Here's how the part is built. I have some questions about the finished solid (model axes, mm). Round coordinates to 2 decimals unless told otherwise and drop trailing zeros. Loops run counter-clockwise (first coordinate to the right, second up) from the corner with the lowest first, then second, coordinate; pieces in that order, holes last. Notation, with made-up numbers: M 83,63.5 L 121,63.5 A22 cw 121,94.5 Z; hole C 58,51 d8. An arc over 180 degrees is marked long. Write each question's results on one line, items separated by ' | '. Start each with the question number.
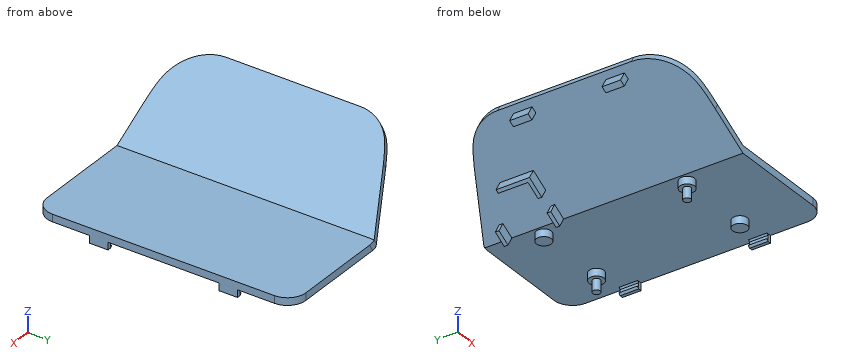
Autodesk Inventor part; units mm, degrees
ref_plane "YZ Plane" through (0, 0, 0) normal (1, 0, 0) x (0, 1, 0)
ref_plane "XZ Plane" through (0, 0, 0) normal (0, 1, 0) x (-1, 0, 0)
ref_plane "XY Plane" through (0, 0, 0) normal (0, 0, 1) x (1, 0, 0)
sketch "スケッチ1" plane through (0, 0, 0) normal (0, 0, 1) x (1, 0, 0)
  line L0 (0, 0) -> (-32, 0)
  line L1 (-32, 0) -> (-32, -70)
  line L2 (-32, -70) -> (0, -70)
  line L3 (0, -70) -> (0, 0)
  dimension "d0" = 32
  dimension "d1" = 70
extrude "押し出し1" add sketch "スケッチ1" along normal blind 2
sketch "スケッチ2" plane through (-32, -70, 0) normal (0, -1, 0) x (1, 0, 0)
  line L0 (0, 0) -> (32, 0)
  line L1 (32, 0) -> (32, 2)
  line L2 (0, 2) -> (32, 2)
  line L3 (0, 0) -> (0, 2)
  line L4 (0, 0) -> (-25.9808, 15)
  line L5 (-25.9808, 15) -> (-25.1147, 16.5)
  line L6 (-25.1147, 16.5) -> (0, 2)
  point P0 (32, 0)
  dimension "d4" = 30
  dimension "d5" = 150
extrude "押し出し2" add sketch "スケッチ2" against normal blind 70 contours L4 L5 L6 L3
sketch "スケッチ3" plane through (0, 0, 0) normal (0, 0, -1) x (-1, 0, 0)
  line L0 (0, 0) -> (32, 0)
  line L1 (32, 0) -> (57.9808, -12.115)
  line L2 (32, 0) -> (57.9808, 0)
  line L3 (57.9808, -70) -> (57.9808, 0)
  dimension "d8" = 25
extrude "押し出し3" cut sketch "スケッチ3" against normal blind 70
sketch "スケッチ4" plane through (0, 0, 0) normal (0, 0, -1) x (-1, 0, 0)
  circle A0 centre (9.1, -14.36) radius 1.15
  circle A1 centre (29.46, -53.14) radius 1.15
  circle A2 centre (9.1, -14.36) radius 1
  circle A3 centre (29.46, -53.14) radius 1
  point P0 (0, 0)
  dimension "d11" = 2
  dimension "d12" = 2
extrude "押し出し4" add sketch "スケッチ4" along normal blind 5 contours A2 | A3
sketch "スケッチ5" plane through (0, 0, 0) normal (0, 0, -1) x (-1, 0, 0)
  circle A0 centre (9.1, -14.36) radius 1
  circle A1 centre (29.46, -53.14) radius 1
  circle A2 centre (9.1, -14.36) radius 2
  circle A3 centre (29.46, -53.14) radius 2
  line L0 (9.1, -14.36) -> (29.46, -14.36)
  line L1 (29.46, -14.36) -> (29.46, -53.14)
  line L2 (29.46, -53.14) -> (9.1, -53.14)
  line L3 (9.1, -53.14) -> (9.1, -14.36)
  circle A4 centre (29.46, -14.36) radius 2
  circle A5 centre (9.1, -53.14) radius 2
  point P0 (0, 0)
  dimension "d15" = 4
  dimension "d16" = 4
  dimension "d17" = 4
  dimension "d18" = 4
extrude "押し出し5" add sketch "スケッチ5" along normal blind 2 contours L0 L3 A0 | L0 A2 L3 A0 | A0 L3 L0 | A0 L3 A2 L0 | A4 L1 L0 | L0 L1 A4 | A5 L2 L3 | L3 L2 A5 | L1 A1 L2 A3 | A3 L2 A1 L1
sketch "スケッチ6" plane through (-32, -70, 0) normal (-0.5, 0, -0.866) x (-0.866, 0, 0.5)
  circle A0 centre (6, 56) radius 4
  line L0 (12, 62) -> (0, 62)
  line L1 (0, 62) -> (0, 50)
  line L2 (0, 50) -> (12, 50)
  line L3 (12, 50) -> (12, 62)
  line L4 (12.5, 62.5) -> (-0.5, 62.5)
  line L5 (-0.5, 62.5) -> (-0.5, 49.5)
  line L6 (-0.5, 49.5) -> (12.5, 49.5)
  line L7 (12.5, 49.5) -> (12.5, 62.5)
  line L8 (13.5, 63.5) -> (-1.5, 63.5)
  line L9 (-1.5, 63.5) -> (-1.5, 48.5)
  line L10 (-1.5, 48.5) -> (13.5, 48.5)
  line L11 (13.5, 48.5) -> (13.5, 63.5)
  line L12 (4, 48.5) -> (8, 48.5)
  line L13 (8, 48.5) -> (8, 49.5)
  line L14 (8, 49.5) -> (4, 49.5)
  line L15 (4, 49.5) -> (4, 48.5)
  line L16 (4, 62.5) -> (8, 62.5)
  line L17 (8, 62.5) -> (8, 63.5)
  line L18 (8, 63.5) -> (4, 63.5)
  line L19 (4, 63.5) -> (4, 62.5)
  line L20 (6, 48.5) -> (6, 63.5)
  line L21 (0, 70) -> (0, 0)
  line L22 (0, 48.5) -> (0, 63.5)
  line L23 (12.5, 57.5369) -> (13.5, 57.5369)
  point P0 (-27.7128, 70)
  point P1 (0, 62.5)
  point P2 (0, 49.5)
  point P3 (4, 49.5)
  dimension "d21" = 0.5
  dimension "d22" = 1
  dimension "d23" = 4
  dimension "d24" = 7.5
  dimension "d25" = 2
extrude "押し出し6" add sketch "スケッチ6" along normal blind 3 contours L21 L8 L19 L4 | L6 L15 L10 L21 | L6 L7 L23 L11 L10 L13
sketch "スケッチ9" plane through (-57.9808, -70, 15) normal (-0.5, 0, -0.866) x (-0.866, 0, 0.5)
  line L0 (-57.7128, 70) -> (-30, 70)
  spline S0 degree 3 poles (-17.6456, 0) (-14.5389, 0) (-12.4319, 0.0723) (-9.2674, 0.5484) (-7.4551, 0.9854) (-4.3314, 2.8768) (-3.1964, 3.9013) (-1.5196, 6.1498) (-0.9279, 7.3003) (-0.1818, 9.6493) (0, 10.8209) (0, 12) knots 0 0 0 0 0.932002 0.932002 1.694801 1.694801 2.239825 2.239825 2.701159 2.701159 3.124298 3.124298 3.124298 3.124298
  spline S1 degree 3 poles (0, 48.1402) (0, 49.6683) (-0.3054, 51.1785) (-1.3061, 53.5747) (-2.0656, 55.0439) (-4.46, 57.4051) (-5.4298, 58.109) (-8.0471, 59.7175) (-9.9104, 60.6321) (-11.1228, 61.1974) knots 0 0 0 0 0.458444 0.458444 0.77844 0.77844 0.966355 0.966355 1.242442 1.242442 1.242442 1.242442
  line L1 (-11.1228, 61.1974) -> (-28.9954, 69.5315)
  line L2 (-11.1228, 61.1974) -> (-28.9954, 69.5315)
  arc A0 (-28.9954, 69.5315) -> (-31.1085, 70) centre (-31.1085, 65) ccw
  line L3 (0, 57.885) -> (-30, 70)
  line L4 (0, 0) -> (0, 57.885)
  line L5 (0, 0) -> (-30, 0)
  line L6 (0, 57.885) -> (0, 70)
  line L7 (0, 70) -> (-31.1085, 70)
  point P0 (-53.3827, 70)
  point P1 (-30, 70)
extrude "押し出し9" cut sketch "スケッチ9" against normal blind 70
sketch "スケッチ10" plane through (-32, -70, 0) normal (-0.5, 0, -0.866) x (-0.866, 0, 0.5)
  spline S0 degree 3 poles (12.3544, 2) (14.3729, 2) (16.0097, 2.0362) (19.2589, 2.3162) (21.0143, 2.657) (23.8072, 4.1137) (24.8109, 4.9066) (26.4147, 6.7969) (27.0131, 7.8518) (27.7245, 9.9614) (27.8914, 10.977) (27.8914, 11.9999) knots 0 0 0 0 0.605548 0.605548 1.419175 1.419175 1.976207 1.976207 2.502247 2.502247 2.949437 2.949437 2.949437 2.949437
  spline S1 degree 3 poles (27.8914, 48.1552) (27.8914, 49.4139) (27.6391, 50.6569) (26.7879, 52.6951) (26.1446, 53.898) (24.1844, 55.8315) (23.3911, 56.4221) (21.0683, 57.9103) (19.2685, 58.8082) (18.0319, 59.3848) knots 0 0 0 0 0.377607 0.377607 0.661941 0.661941 0.825328 0.825328 1.114005 1.114005 1.114005 1.114005
  line L0 (27.8981, 15.078) -> (26.2914, 15.078)
  line L1 (26.2914, 15.078) -> (26.2914, 20.078)
  line L2 (26.2914, 20.078) -> (27.8981, 20.078)
  line L3 (27.8981, 20.078) -> (27.8981, 15.078)
  line L4 (27.8981, 15.078) -> (27.9914, 15.078)
  line L5 (27.9914, 15.078) -> (27.9914, 20.078)
  line L6 (27.9914, 20.078) -> (27.8981, 20.078)
  line L7 (27.8981, 20.078) -> (27.8981, 15.078)
  spline S2 degree 3 poles (12.3544, 2) (14.3729, 2) (16.0097, 2.0362) (19.2589, 2.3162) (21.0143, 2.657) (23.8072, 4.1137) (24.8109, 4.9066) (26.4147, 6.7969) (27.0131, 7.8518) (27.7245, 9.9614) (27.8914, 10.977) (27.8914, 11.9999) knots 0 0 0 0 0.605548 0.605548 1.419175 1.419175 1.976207 1.976207 2.502247 2.502247 2.949437 2.949437 2.949437 2.949437
  spline S3 degree 3 poles (27.8914, 48.1552) (27.8914, 49.4139) (27.6391, 50.6569) (26.7879, 52.6951) (26.1446, 53.898) (24.1844, 55.8315) (23.3911, 56.4221) (21.0683, 57.9103) (19.2685, 58.8082) (18.0319, 59.3848) knots 0 0 0 0 0.377607 0.377607 0.661941 0.661941 0.825328 0.825328 1.114005 1.114005 1.114005 1.114005
  line L8 (30, 12) -> (30, 48.1402)
  line L9 (27.9457, 30.078) -> (29.9457, 30.078)
  line L10 (27.8981, 45.078) -> (26.2914, 45.078)
  line L11 (26.2914, 45.078) -> (26.2914, 40.078)
  line L12 (26.2914, 40.078) -> (27.8981, 40.078)
  line L13 (27.8981, 40.078) -> (27.8981, 45.078)
  line L14 (27.8981, 45.078) -> (27.9914, 45.078)
  line L15 (27.9914, 45.078) -> (27.9914, 40.078)
  line L16 (27.9914, 40.078) -> (27.8981, 40.078)
  line L17 (27.8981, 40.078) -> (27.8981, 45.078)
  line L18 (27.8914, 22.078) -> (27.8914, 38.078)
  point P0 (-27.7128, 70)
  point P1 (30, 48.1402)
  point P2 (28.9457, 30.078)
  point P3 (27.0948, 15.078)
  point P4 (27.0948, 45.078)
  point P5 (27.8981, 40.078)
  dimension "d34" = 5
  dimension "d38" = 5
  dimension "d55" = 15
  dimension "d58" = 0.1
  dimension "d59" = 1.6
  dimension "d60" = 8
  dimension "d61" = 2
extrude "押し出し10" add sketch "スケッチ10" along normal blind 3
sketch "スケッチ11" plane through (0, 0, 0) normal (0, 0, -1) x (-1, 0, 0)
  line L0 (0, 0) -> (0, -64.8508)
  line L1 (0, -20) -> (0.9, -20)
  line L2 (0.9, -20) -> (0.9, -15)
  line L3 (0.9, -15) -> (0, -15)
  line L4 (0, -15) -> (0, -20)
  line L5 (0, -35) -> (4.5878, -35)
  line L6 (0, -50) -> (0.9, -50)
  line L7 (0.9, -50) -> (0.9, -55)
  line L8 (0.9, -55) -> (0, -55)
  line L9 (0, -55) -> (0, -50)
  line L10 (0, 0) -> (29.5653, 0)
  line L11 (0, -70) -> (0, 0)
  point P0 (0, -50)
  point P1 (0, -55)
  point P2 (0, -15)
  dimension "d41" = 5
  dimension "d42" = 15
  dimension "d43" = 0.9
  dimension "d62" = 35
extrude "押し出し11" add sketch "スケッチ11" along normal blind 2
sketch "スケッチ12" plane through (-0.9, -55, 0) normal (0, -1, 0) x (1, 0, 0)
  line L0 (0, 0) -> (0.9, 0)
  line L1 (0, 0) -> (0, -2)
  line L2 (0.9, -2) -> (0, -2)
  line L3 (0.9, 0) -> (0.9, -2)
  line L4 (0, -2) -> (-0.5, -2)
  line L5 (-0.5, -2) -> (-0.5, -1.5)
  line L6 (-0.5, -1.5) -> (0, -1.5)
  line L7 (0, -1.5) -> (0, -2)
  line L8 (0, -2) -> (-0.5, -1.5)
  point P0 (0.9, 0)
  point P1 (0, -1.5)
  dimension "d46" = 0.5
  dimension "d47" = 0.5
extrude "押し出し12" add sketch "スケッチ12" against normal blind 5 contours L1 L8 L6
sketch "スケッチ13" plane through (-0.9, -20, 0) normal (0, -1, 0) x (1, 0, 0)
  line L0 (0, 0) -> (0.9, 0)
  line L1 (0, 0) -> (0, -1.5)
  line L2 (0, -1.5) -> (-0.5, -1.5)
  line L3 (-0.5, -1.5) -> (0, -2)
  line L4 (0.9, -2) -> (0, -2)
  line L5 (0.9, 0) -> (0.9, -2)
  line L6 (0, -2) -> (0, -1.5)
  point P0 (0.9, 0)
extrude "押し出し13" add sketch "スケッチ13" against normal blind 5 contours L6 L3 L2
chamfer "面取り1" distance 0.4 angle 45 2 edges at (-0.9, -17.5, 0) (-0.9, -52.5, 0)
fillet "フィレット1" radius 5 2 edges at (0, -70, 1) (0, 0, 1)
properties part number "case"
1. I want a section at A-A on x = -9.1. List the corners of the cut face in (y, z) for me, plus the area to 3 significant figures.
2. I want a section at B-B on y = -53.14. List the corners of the cut face in (x, z) for me, plus the area to 3 significant figures.
3. I want a section at D-D on x = -22.5. List the corners of the cut face in (y, z) for me, plus the area to 3 significant figures.
4. For pin 1 (2.5 mm diameter, centred on x = -35.5, z = -0.5, fed in from +Y); pin 2 (5 mm diameter, centred on x = -31.5, y = -56.5, fed in from -Z); pin 3 (0.6 mm diameter, centred on x = -1, z = -1.5, fed in from +Y); pin 4 (2 mm diameter, centred on y = -25, z = 0, fed in from +X), each with a flat end and sliding along its axis, tell me the tip position at first contact or that it passes through.
5. I want a section at C-C on y = -46. List the corners of the cut face in (x, z) for me, plus the area to 3 significant figures.
6. I need wall thicknesses on line 1 along X through (y, z) = (-52, -1.75); line 2 along Z through (x, y) = (-6, -50); line 3 along X through (y, z) = (-12.5, 5.25). Which ranges of each line are inside material? Lowest first, please.
Outcome:
1) outline: M -70,0 L -55.14,0 L -55.14,-2 L -51.14,-2 L -51.14,0 L -16.36,0 L -16.36,-2 L -15.36,-2 L -15.36,-5 L -13.36,-5 L -13.36,-2 L -12.36,-2 L -12.36,0 L 0,0 L 0,2 L -70,2 Z | area: 162 mm2
2) outline: M -57.98,15 L -56.24,14 L -57.74,11.4 L -56.27,10.55 L -54.77,13.15 L -32,0 L -31.46,0 L -31.46,-2 L -30.46,-2 L -30.46,-5 L -28.46,-5 L -28.46,-2 L -27.46,-2 L -27.46,0 L -11.1,0 L -11.1,-2 L -7.1,-2 L -7.1,0 L -1.3,0 L -0.9,-0.4 L -0.9,-1.5 L -1.4,-1.5 L -0.9,-2 L 0,-2 L 0,2 L -32,2 L -57.11,16.5 Z | area: 144 mm2
3) outline: M -70,0 L 0,0 L 0,2 L -70,2 Z | area: 140 mm2
4) pin 1: y = -6.5 | pin 2: z = -2 | pin 3: y = -15 | pin 4: x = 0
5) outline: M -57.98,15 L -32,0 L 0,0 L 0,2 L -32,2 L -57.11,16.5 Z | area: 115 mm2
6) line 1: -31.1 to -27.82, -10.74 to -7.46, -1.15 to 0 | line 2: 0 to 2 | line 3: -44.56 to -43.4, -41.09 to -37.63
